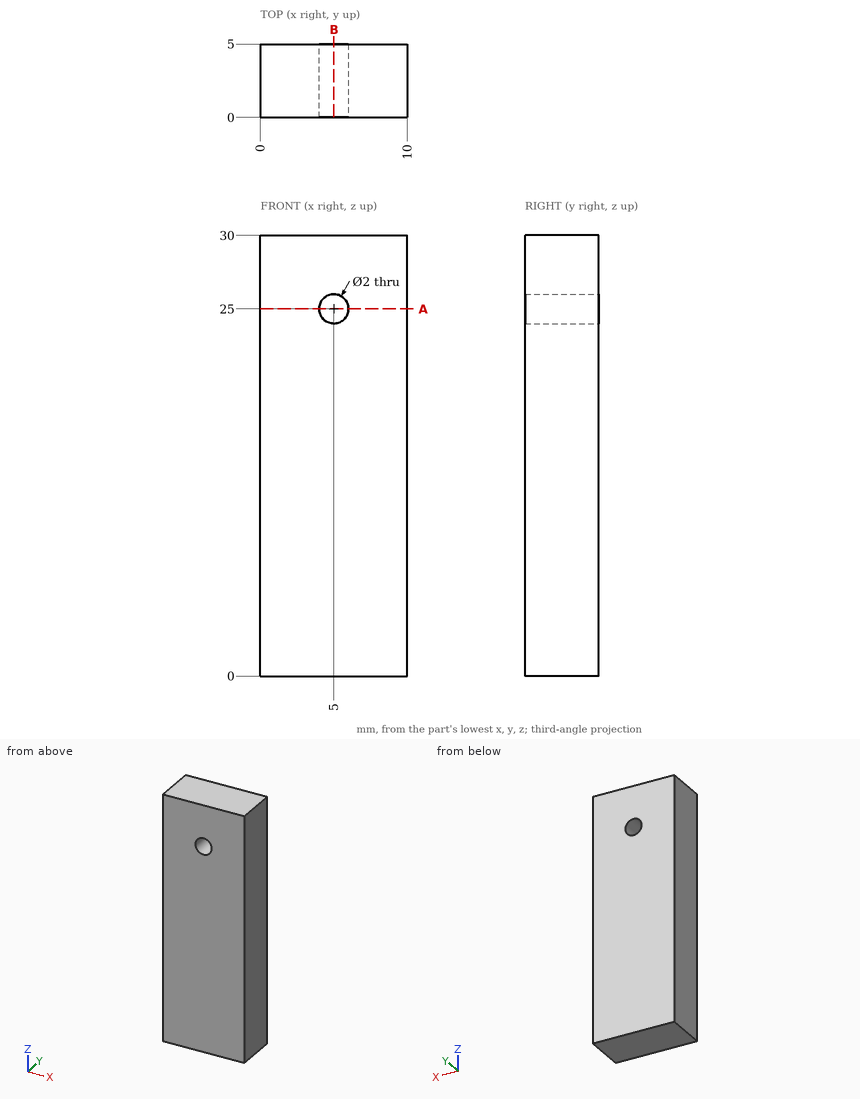
The drawing under review shows one solid part. Ordinate dimensions are in mm from its lowest x, y, z. Coordinates: 2 decimals unless noted, no trailing zeros. Loops run counter-clockwise (first coordinate to the right, second up) from the corner with the lowest first, then second, coordinate; pieces in that order, holes last. Notation, with made-up numbers: (62.5, 75.25) -> (84.5, 75.25) arc R37 ccw to (84.5, 113.25) -> close; hole circle Ø9 at (2.5, 31). An arc over 180 degrees is marked (long way). Answer as a JSON object with one key per item and string values.
Q1. To check wall thickness, follow L1, parallel to Z at x = 5, y = 0.4; L2, parallel to X at y = 1.2, z = 25; L3, parallel to X at y = 2.9, z = 24.25. State the ranges of each line that lie inside material, in increasing order.
Answer block:
{"L1": "z = 0 to 24, 26 to 30", "L2": "x = 0 to 4, 6 to 10", "L3": "x = 0 to 4.34, 5.66 to 10"}
Q2. Take a section at B-B on x = 5. Give the boundary of the cut face in (y, z), plus the area to 3 significant figures.
Answer block:
{"outline": "(0, 0) -> (5, 0) -> (5, 24) -> (0, 24) -> close; (0, 26) -> (5, 26) -> (5, 30) -> (0, 30) -> close", "area": "140 mm^2"}
Q3. Take a section at A-A on z = 25. Give the boundary of the cut face in (x, y).
Answer block:
{"outline": "(0, 0) -> (4, 0) -> (4, 5) -> (0, 5) -> close; (6, 0) -> (10, 0) -> (10, 5) -> (6, 5) -> close"}
